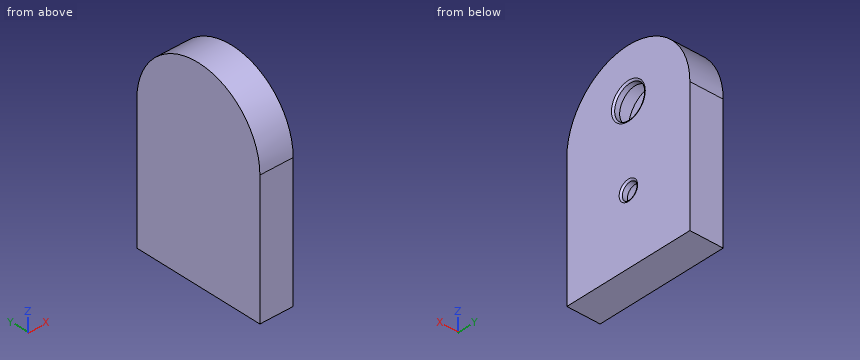
```python
from build123d import *

# Parameters (mm, degrees)
F1_DEPTH = 40
F2_R     = 37.5
F2_R_2   = 20
F4_DEPTH = 25
F5_R     = 12.5
F5_R_2   = 25
F6_DEPTH = 10
F7_R     = 2.5


with BuildPart() as f1:
    # F0 (on Right) → F1 (new body)
    with BuildSketch(Plane.YZ):
        with BuildLine():
            Line((-100, -100), (100, -100))
            Line((100, -100), (100, 100))
            ThreePointArc((100, 100), (0, 200), (-100, 100))
            Line((-100, 100), (-100, -100))
        make_face()
    extrude(amount=F1_DEPTH)

    # F2 (on face) → F4 (cut)
    with BuildSketch(Plane.YZ.offset(40)):
        with Locations((0, 125)):
            Circle(F2_R)
        with Locations((0, 5)):
            Circle(F2_R_2)
    extrude(amount=-F4_DEPTH, mode=Mode.SUBTRACT)

    # F5 (on face) → F6 (join)
    with BuildSketch(Plane.YZ.offset(40)):
        with BuildLine():
            Line((-100, -100), (100, -100))
            Line((100, -100), (100, 100))
            ThreePointArc((100, 100), (0, 200), (-100, 100))
            Line((-100, 100), (-100, -100))
        make_face()
        with Locations((0, 5)):
            Circle(F5_R, mode=Mode.SUBTRACT)
        with Locations((0, 125)):
            Circle(F5_R_2, mode=Mode.SUBTRACT)
    extrude(amount=F6_DEPTH)

    # F7
    f7_edges = [f1.edges().sort_by_distance(p)[0] for p in [
        (50, -25, 125),
        (50, -12.5, 5),
    ]]
    fillet(f7_edges, radius=F7_R)


solid = f1.part
```
The model under review builds one solid part; all positions refer to its coordinate system, in mm. Round coordinates to 2 decimals unless told otherwise and drop trailing zeros. Order: outer loops, then holes, each group sorted by start corner. A loop starts at its lowest first (then second) coordinate and runs counter-clockwise, first axis right, second up. Notation, with made-up numbers: (15, 23) -> (20, 23) arc R26 cw to (20, 37) -> close; hole circle Ø6 at (23.25, 71.5). An arc over 180 degrees is marked (long way). Use a Markdown table: item, result.
Q1. For line 1 (Z direction, x = 42.5, y = 0); line 2 (Z direction, x = 30.5, y = 0); line 3 (Y direction, x = 19, z = 11), list the stretches that pass through material, from the lowest coordinate up.
Values:
| item | result |
|---|---|
| line 1 | z = -100 to -7.5, 17.5 to 100, 150 to 200 |
| line 2 | z = -100 to -15, 25 to 87.5, 162.5 to 200 |
| line 3 | y = -100 to -19.08, 19.08 to 100 |
Q2. Clearance check with flat-ended pins moving along their axes: P1, Ø2, axis at x = 30, y = -67.5, coming from the +Z side; P2, Ø3, axis at y = 21, z = 136, coming from the +X side (3 decimals); P3, Ø5, axis at x = 29.5, y = 4.5, coming from the +Z side. State where each tip first meets the part, or that it passes through.
Values:
| item | result |
|---|---|
| P1 | stops at z = 174.68 |
| P2 | stops at x = 48.495 |
| P3 | stops at z = 199.98 |
Q3. We need section C-C on z = 125. Write out the cut boundary in (x, y).
Values:
| item | result |
|---|---|
| outline | (0, -96.82) -> (50, -96.82) -> (50, -27.5) arc R2.5 ccw to (47.5, -25) -> (40, -25) -> (40, -37.5) -> (15, -37.5) -> (15, 37.5) -> (40, 37.5) -> (40, 25) -> (47.5, 25) arc R2.5 ccw to (50, 27.5) -> (50, 96.82) -> (0, 96.82) -> close |
Q4. We need section D-D on y = 64.5. Write out the cut boundary in (x, z).
Values:
| item | result |
|---|---|
| outline | (0, -100) -> (50, -100) -> (50, 176.42) -> (0, 176.42) -> close |
Q5. We need section A-A on x = 25. Write out the cut boundary in (y, z), then the cut area to 3 significant figures.
Values:
| item | result |
|---|---|
| outline | (-100, -100) -> (100, -100) -> (100, 100) arc R100 ccw to (-100, 100) -> close; hole circle Ø75 at (0, 125); hole circle Ø40 at (0, 5) |
| area | 50,000 mm^2 |
Q6. We need section B-B on y = 0. Write out the cut boundary in (x, z), then the cut area to 3 significant figures.
Values:
| item | result |
|---|---|
| outline | (0, -100) -> (50, -100) -> (50, -10) arc R2.5 ccw to (47.5, -7.5) -> (40, -7.5) -> (40, -15) -> (15, -15) -> (15, 25) -> (40, 25) -> (40, 17.5) -> (47.5, 17.5) arc R2.5 ccw to (50, 20) -> (50, 97.5) arc R2.5 ccw to (47.5, 100) -> (40, 100) -> (40, 87.5) -> (15, 87.5) -> (15, 162.5) -> (40, 162.5) -> (40, 150) -> (47.5, 150) arc R2.5 ccw to (50, 152.5) -> (50, 200) -> (0, 200) -> close |
| area | 11,400 mm^2 |
